The listing builds one solid part. Answer for the finished solid, in the listing's coordinates (mm). A direction names the side the tool comes from. Round coordinates to 2 decimals unless told otherwise and drop trailing zeros. Write each loop counter-clockwise with the first axis right and the second up, starting at its lowest first coordinate (ties: lowest second). Pieces come first, ordered by that corner, then holes.
(1) A cutting plane is placed at B-B, the plane x = -34. Give the vertices of the cut face in (y, z).
(2) For faces 1 (the face through (-22, 9, -32.529)), 2 (the face through (-28.03, 7.99, 42.23)), 3 (the face through (-30.498, 9, -26)), determine the directions among +Z, -Z, +X, -X, +Y, -Y from which every point of the face is accessible in a straight line to the end or side of a thin tool.
(3) A cutting plane is placed at D-D, the plane z = -22. Give the vertices of the cut face in (x, y).
(4) A cutting plane is placed at C-C, the plane y = 17.25. Give the vertices of the cut face in (x, z).
(5) A cutting plane is placed at A-A, the plane x = -21. Give the vertices of the cut face in (y, z), and give its area (3 significant figures).
(6) Each of these flat-tipped pins is pushed along its axis until it touches: pin 1 Ø1.5 at (x, y) = (-41, 14) entering from -Z; pin 2 Ø1 at (y, z) = (6, 6) entering from -X; pin 3 Ø5 at (y, z) = (12.5, 26.5) entering from +X; pin 4 Ø12 at (x, z) = (-39.5, 34.5) entering from -Y. Where does it stop, or does it pass through?
(7) Find the intervals of material crossed by probe 1 along Y at (x, z) = (-19.5, -29); probe 2 along Z at (x, y) = (-24, 8); probe 3 along Y at (x, z) = (-30, 44.5), in increasing order.
(8) The mould has two halves that part along Z. Classify faces 4 (the face through (-30.498, 9, 40)), 5 (the face through (-14.491, 13.019, 37.735)), 6 (the face through (-44.995, 8.874, 7.033)): +Z half, -Z half, draft (parallel to the pull), parting line (faces both ways), or undercut.
from build123d import *

# Parameters (mm, degrees)
BOSS_EXTRUDE1_DEPTH = 18
SKETCH2_R           = 1.75
CUT_EXTRUDE1_DEPTH  = 32
CUT_EXTRUDE2_DEPTH  = 1
CUT_EXTRUDE3_DEPTH  = 5


with BuildPart() as part:
    # Sketch1 → Boss-Extrude1 (new body)
    with BuildSketch(Plane(origin=(0, 0, 0), x_dir=(1, 0, 0), z_dir=(0, 1, 0))):
        with BuildLine():
            Line((-13.998275301, 32.528571429), (-30.498275301, 32.528571429))
            Line((-30.498275301, 32.528571429), (-30.498275301, 18.772618373))
            ThreePointArc((-30.498275301, 18.772618373), (-22.584151632, 22.315862806), (-13.998275301, 23.528571429))
            Line((-13.998275301, 23.528571429), (-13.998275301, 32.528571429))
        make_face()
        with BuildLine():
            ThreePointArc((-13.998275301, 23.528571429), (-22.584151632, 22.315862806), (-30.498275301, 18.772618373))
            ThreePointArc((-30.498275301, 18.772618373), (-44.998275301, -7.471428571), (-30.498275301, -33.715475515))
            ThreePointArc((-30.498275301, -33.715475515), (-22.584151632, -37.258719949), (-13.998275301, -38.471428571))
            Line((-13.998275301, -38.471428571), (-13.998275301, -31.471428571))
            ThreePointArc((-13.998275301, -31.471428571), (-37.998275301, -7.471428571), (-13.998275301, 16.528571429))
            Line((-13.998275301, 16.528571429), (-13.998275301, 23.528571429))
        make_face()
        with BuildLine():
            Line((-30.498275301, -33.715475515), (-30.498275301, -47.471428571))
            Line((-30.498275301, -47.471428571), (-13.998275301, -47.471428571))
            Line((-13.998275301, -47.471428571), (-13.998275301, -38.471428571))
            ThreePointArc((-13.998275301, -38.471428571), (-22.584151632, -37.258719949), (-30.498275301, -33.715475515))
        make_face()
    extrude(amount=BOSS_EXTRUDE1_DEPTH)

    # Sketch2 → Cut-Extrude1 (cut, through all)
    with BuildSketch(Plane(origin=(-13.998275301, 0, 0), x_dir=(0, 0, -1), z_dir=(1, 0, 0))):
        with Locations((-42.471428571, 5.25)):
            Circle(SKETCH2_R)
        with Locations((27.528571429, 5.25)):
            Circle(SKETCH2_R)
    extrude(amount=-CUT_EXTRUDE1_DEPTH, mode=Mode.SUBTRACT)

    # Sketch3 → Cut-Extrude2 (cut)
    with BuildSketch(Plane(origin=(-13.998275301, 0, 0), x_dir=(0, 0, -1), z_dir=(1, 0, 0))):
        Polygon((-41.872123333, 14.596956651), (-39.29413188, 14.596956651), (-39.29413188, 13.647170326), (-40.922337009, 13.647170326), (-40.922337009, 12.629542121), (-39.29413188, 12.629542121), (-39.29413188, 11.679755796), (-40.922337009, 11.679755796), (-40.922337009, 9.305289984), (-41.872123333, 9.305289984), align=None)
        Polygon((-36.619677754, 14.732640412), (-35.630670342, 14.732640412), (-35.630670342, 11.272704514), (-35.15577718, 11.272704514), (-35.15577718, 10.39076007), (-35.630670342, 10.39076007), (-35.630670342, 9.305289984), (-36.580456667, 9.305289984), (-36.580456667, 10.39076007), (-38.819238718, 10.39076007), (-38.819238718, 11.352206718), align=None)
        Polygon((-36.580456667, 11.272704514), (-36.580456667, 13.073694431), (-37.751789132, 11.272704514), align=None, mode=Mode.SUBTRACT)
    extrude(amount=-CUT_EXTRUDE2_DEPTH, mode=Mode.SUBTRACT)

    # Sketch4 → Cut-Extrude3 (cut)
    with BuildSketch(Plane.ZY.offset(30.498275301)):
        Polygon((-25.218846283, 3.070893971), (-24.486547677, 6.160727637), (-26.796272822, 8.339833666), (-29.838296574, 7.429106029), (-30.57059518, 4.339272363), (-28.260870035, 2.160166334), align=None)
        Polygon((44.316873767, 2.665882092), (45.632062924, 5.556143466), (43.786617729, 8.140261375), (40.625983376, 7.834117908), (39.310794219, 4.943856534), (41.156239414, 2.359738625), align=None)
    extrude(amount=-CUT_EXTRUDE3_DEPTH, mode=Mode.SUBTRACT)


solid = part.part
Solutions:
1. outline: (0, -16.21) - (18, -16.21) - (18, -5.79) - (0, -5.79) - close; (0, 20.74) - (18, 20.74) - (18, 31.16) - (0, 31.16) - close
2. face 1: -Z, +X, -X, +Y, -Y
2. face 2: -X
2. face 3: -Z, -X, +Y, -Y
3. outline: (-30.5, 0) - (-14, 0) - (-14, 18) - (-30.5, 18) - close
4. outline: (-30.5, -32.53) - (-14, -32.53) - (-14, -16.53) arc R24 cw to (-14, 31.47) - (-14, 47.47) - (-30.5, 47.47) - (-30.5, 33.72) arc R31 ccw to (-30.5, -18.77) - close
5. outline: (0, -32.53) - (18, -32.53) - (18, -15.48) - (0, -15.48) - close; (0, 30.43) - (18, 30.43) - (18, 47.47) - (0, 47.47) - close; hole circle Ø3.5 at (5.25, -27.53); hole circle Ø3.5 at (5.25, 42.47)
5. area: 594 mm2
6. pin 1: stops at z = -9.02
6. pin 2: stops at x = -44.98
6. pin 3: stops at x = -24.61
6. pin 4: passes through
7. probe 1: y = 0 to 4.3, 6.2 to 18
7. probe 2: z = -32.53 to -14.35, 29.29 to 47.47
7. probe 3: y = 0 to 3.07, 7.14 to 18
8. face 4: draft
8. face 5: undercut
8. face 6: parting line
